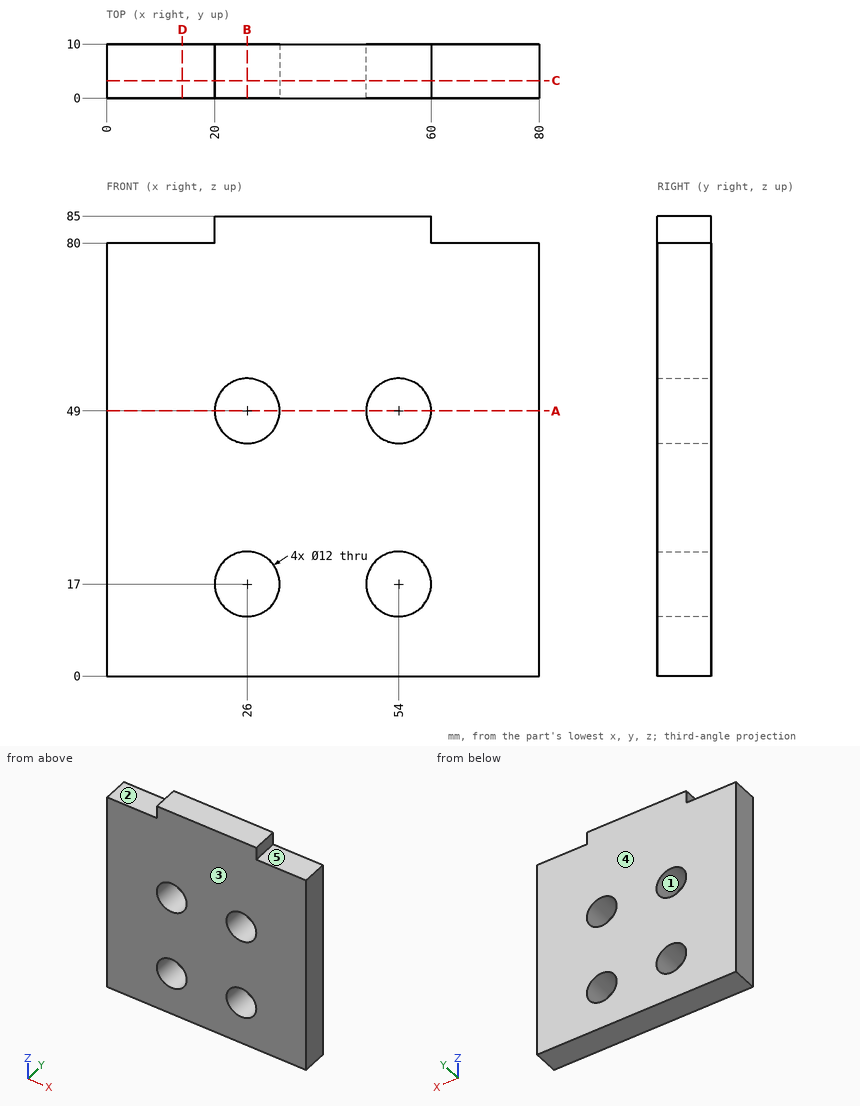
Study the drawing (mm; zero at the part's minimum x, y, z) and answer. A direction names the side the tool comes from. Give positions to 0.01 mm unless a question says otherwise; leave off trailing zeros. Write each loop counter-clockwise with the first axis right and the second up, starting at its lowest first coordinate (ties: lowest second). Pieces come first, ordered by that corner, then holes. Notation, with made-up numbers: (-36, -14) -> (-30, -14) arc R28 cw to (-30, 23) -> close; hole circle Ø2 at (32.5, -12.5). An arc over 180 degrees is marked (long way). Write item = value, one per line.
Q1. Section D-D on x = 14 is taken. Determine the outline of the cut face in (y, z).
Computed values:
outline = (0, 0) -> (10, 0) -> (10, 80) -> (0, 80) -> close
Q2. Section A-A on z = 49 is taken. Determine the outline of the cut face in (x, y), and give its area (3 significant figures).
Computed values:
outline = (0, 0) -> (20, 0) -> (20, 10) -> (0, 10) -> close; (32, 0) -> (48, 0) -> (48, 10) -> (32, 10) -> close; (60, 0) -> (80, 0) -> (80, 10) -> (60, 10) -> close
area = 560 mm^2
Q3. Section C-C on y = 3.25 is taken. Determine the outline of the cut face in (x, z).
Computed values:
outline = (0, 0) -> (80, 0) -> (80, 80) -> (60, 80) -> (60, 85) -> (20, 85) -> (20, 80) -> (0, 80) -> close; hole circle Ø12 at (26, 17); hole circle Ø12 at (26, 49); hole circle Ø12 at (54, 17); hole circle Ø12 at (54, 49)
Q4. Section B-B on x = 26 is taken. Determine the outline of the cut face in (y, z), and give its area (3 significant figures).
Computed values:
outline = (0, 0) -> (10, 0) -> (10, 11) -> (0, 11) -> close; (0, 23) -> (10, 23) -> (10, 43) -> (0, 43) -> close; (0, 55) -> (10, 55) -> (10, 85) -> (0, 85) -> close
area = 610 mm^2
Q5. Consider line 1 along Z through (x, y) = (26, 6); line 2 along Z through (x, y) = (55, 6.75); line 3 along X through (y, z) = (6.5, 47.5). Determine where each line is inside the solid, lowest interval first.
Computed values:
line_1 = 0 to 11, 23 to 43, 55 to 85
line_2 = 0 to 11.08, 22.92 to 43.08, 54.92 to 85
line_3 = 0 to 20.19, 31.81 to 48.19, 59.81 to 80
Q6. A tool of negligible diameter and unlimited length cuts with its end or side. For the marked faces 4 and 5, from which of +Z, -Z, +X, -X, +Y, -Y can it reach the whole face along a straight path? Write none if from no direction.
Computed values:
face_4 = +Z, -Z, +X, -X, +Y
face_5 = +Z, +X, +Y, -Y
Q7. Flat-ended cylindrical pins translate along their axes: pin 1 Ø4 at (y, z) = (4, 82.5) entering from +X; pin 2 Ø4 at (x, y) = (72, 2.5) entering from +Z. Find the tip coordinate at first contact, or state that the pin passes through.
Computed values:
pin_1 = 60
pin_2 = 80
Q8. For a pull along Z with two mould halves and no side action, classify the marked faces 1, 2 and 3 as pulls with the +Z half, pulls with the -Z half, needs draft (parallel to the pull), parting line crosses it, or undercut.
Computed values:
face_1 = undercut
face_2 = pulls with the +Z half
face_3 = needs draft
